Read the model definition and answer for the solid it produces. Units are mm, in the model's axes. Face numbers are marked on the shaded views. A direction names the side the tool comes from. Coordinates: 2 decimals unless noted, no trailing zeros. Loops run counter-clockwise (first coordinate to the right, second up) from the corner with the lowest first, then second, coordinate; pieces in that order, holes last.
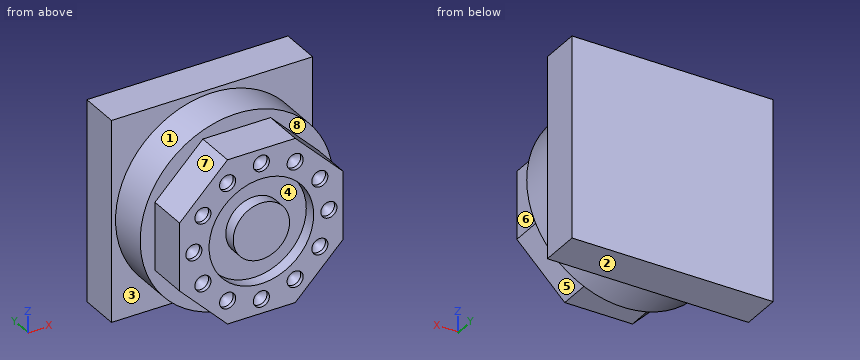
from build123d import *

# Parameters (mm, degrees)
F0_W     = 50
F0_H     = 50
F1_DEPTH = 10
F2_R     = 24
F3_DEPTH = 10
F5_DEPTH = 10
F7_D     = 4
F7_DEPTH = 1
F7_TIP   = 1.2017212381
F8_R     = 13
F8_R_2   = 7
F9_DEPTH = 3


with BuildPart() as f1:
    # F0 (on Front) → F1 (new body)
    with BuildSketch(Plane.XZ):
        Rectangle(F0_W, F0_H)
    extrude(amount=F1_DEPTH)

    # F2 (on face) → F3 (join)
    with BuildSketch(Plane.XZ.offset(10)):
        Circle(F2_R)
    extrude(amount=F3_DEPTH)

    # F4 (on face) → F5 (join)
    with BuildSketch(Plane.XZ.offset(20)):
        Polygon((20.325, 8.4188906552), (8.4188906552, 20.325), (0, 20.325), (-8.4188906552, 20.325), (-20.325, 8.4188906552), (-20.325, -8.4188906552), (-8.4188906552, -20.325), (8.4188906552, -20.325), (20.325, -8.4188906552), align=None)
    extrude(amount=F5_DEPTH)

    # F7
    with Locations(Plane.XZ.offset(30)):
        with Locations((-8.3919226456, 14.5352363953), (0, 16.7838452912), (8.3919226456, 14.5352363953), (14.5352363953, 8.3919226456), (16.7838452912, 0), (14.5352363953, -8.3919226456), (8.3919226456, -14.5352363953), (0, -16.7838452912), (-8.3919226456, -14.5352363953), (-14.5352363953, -8.3919226456), (-16.7838452912, 0), (-14.5352363953, 8.3919226456)):
            Hole(F7_D / 2, depth=F7_DEPTH)
            with Locations((0, 0, -(F7_DEPTH + F7_TIP / 2))):  # 118° drill point
                Cone(0, F7_D / 2, F7_TIP, mode=Mode.SUBTRACT)

    # F8 (on face) → F9 (cut)
    with BuildSketch(Plane.XZ.offset(30)):
        Circle(F8_R)
        Circle(F8_R_2, mode=Mode.SUBTRACT)
    extrude(amount=-F9_DEPTH, mode=Mode.SUBTRACT)


solid = f1.part
Q1. Which of the six approach directions +Z, -Z, +X, -X, +Y, -Y give full straight-line access (tool end or side, diameter ignored) to the marked faces 5, 6, 7 and 8?
Findings below:
face 5: -Z, +X, -Y
face 6: +Z, -Z, +X, -Y
face 7: +Z, -X, -Y
face 8: -Y
Q2. Determine the mould class of the marked faces 1, 2, 3 and 4 for opening direction Z: +Z half, -Z half, draft (parallel to the pull), parting line (faces both ways), or undercut.
Findings below:
face 1: parting line
face 2: -Z half
face 3: draft
face 4: undercut
Q3. Flat-ended cylindrical pins translate along their axes: pin 1 Ø11 at (y, z) = (-27, 3) entering from +X (3 decimals); pin 2 Ø2 at (y, z) = (-11.5, -6.5) entering from +X; pin 3 Ø10 at (x, y) = (-8, -23.5) entering from -Z. Find the tip coordinate at first contact, or state that the pin passes through.
Findings below:
pin 1: stops at x = 20.325
pin 2: stops at x = 23.36
pin 3: stops at z = -23.59
Q4. A cutting plane is placed at B-B (y = -18.25). Give the vertices of the cut face in (x, z).
Findings below:
outline: circle Ø48 at (0, 0)
Q5. Straight lines are drawn through the part: probe 1 along Y at (x, z) = (11, 21.5); probe 2 along Y at (x, z) = (10, 20); probe 3 along X at (y, z) = (-24.25, -2) (3 decimals). For each, find the intervals that lie inside material, in ascending order.
Findings below:
probe 1: y = -10 to 0
probe 2: y = -20 to 0
probe 3: x = -20.325 to 20.325
Q6. A cutting plane is placed at A-A (z = 5.5). Give the vertices of the cut face in (x, y) (3 decimals), then the cut area to 3 significant figures.
Findings below:
outline: (-25, -10) - (-23.361, -10) - (-23.361, -20) - (-20.325, -20) - (-20.325, -30) - (-11.779, -30) - (-11.779, -27) - (-4.33, -27) - (-4.33, -30) - (4.33, -30) - (4.33, -27) - (11.779, -27) - (11.779, -30) - (20.325, -30) - (20.325, -20) - (23.361, -20) - (23.361, -10) - (25, -10) - (25, 0) - (-25, 0) - close
area: 1,330 mm2
